The listing builds one solid part. Answer for the finished solid, in the listing's coordinates (mm). A direction names the side the tool comes from. Give positions to 0.01 mm unless a question says otherwise; leave off trailing zeros. Write each loop counter-clockwise with the first axis right and the second up, starting at its lowest first coordinate (ties: lowest second). Pieces come first, ordered by that corner, then holes. Notation, with made-up numbers: (-26, 79.25) - (-1, 79.25) arc R28 cw to (-1, 101.25) - close; hole circle Ø7 at (22.5, 24). An arc over 180 degrees is marked (long way). One line per item, written item: value. Start each with the question number.
Autodesk Inventor part; units mm, degrees
ref_plane "YZ Plane" through (0, 0, 0) normal (1, 0, 0) x (0, 1, 0)
ref_plane "XZ Plane" through (0, 0, 0) normal (0, 1, 0) x (-1, 0, 0)
ref_plane "XY Plane" through (0, 0, 0) normal (0, 0, 1) x (1, 0, 0)
sketch "Sketch1" plane through (0, 0, 0) normal (0, 0, 1) x (1, 0, 0)
  line L0 (127, 0) -> (127, 203.2)
  line L1 (127, 203.2) -> (0, 203.2)
  line L2 (0, 203.2) -> (0, 0)
  line L3 (95.25, 0) -> (95.25, 184.15)
  line L4 (95.25, 184.15) -> (31.75, 184.15)
  line L5 (31.75, 184.15) -> (31.75, 0)
  line L6 (0, 0) -> (31.75, 0)
  line L7 (95.25, 0) -> (127, 0)
  circle A0 centre (6.35, 6.35) radius 3.175
  circle A1 centre (120.65, 6.35) radius 3.175
  circle A2 centre (6.35, 196.85) radius 3.175
  circle A3 centre (120.65, 196.85) radius 3.175
  circle A4 centre (9.525, 101.6) radius 1.5875
  circle A5 centre (25.4, 101.6) radius 1.5875
  circle A6 centre (9.525, 76.2) radius 1.5875
  circle A7 centre (25.4, 76.2) radius 1.5875
extrude "Extrusion1" add sketch "Sketch1" along normal blind 15.875
chamfer "Chamfer1" distance 3.175 angle 45 2 edges at (31.75, 0, 7.9375) (95.25, 0, 7.9375)
fillet "Fillet1" radius 3.175 2 edges at (31.75, 184.15, 7.9375) (95.25, 184.15, 7.9375)
sketch "Sketch2" plane through (0, 0, 15.875) normal (0, 0, 1) x (1, 0, 0)
  arc A0 (6.35, 190.5) -> (12.7, 196.85) centre (6.35, 196.85) ccw
  line L0 (12.7, 196.85) -> (12.7, 203.2)
  line L1 (12.7, 203.2) -> (0, 203.2)
  line L2 (0, 203.2) -> (0, 190.5)
  line L3 (0, 190.5) -> (6.35, 190.5)
  arc A1 (114.3, 196.85) -> (120.65, 190.5) centre (120.65, 196.85) ccw
  line L4 (114.3, 196.85) -> (114.3, 203.2)
  line L5 (114.3, 203.2) -> (127, 203.2)
  line L6 (127, 203.2) -> (127, 190.5)
  line L7 (127, 190.5) -> (120.65, 190.5)
  arc A2 (12.7, 6.35) -> (6.35, 12.7) centre (6.35, 6.35) ccw
  line L8 (6.35, 12.7) -> (0, 12.7)
  line L9 (0, 12.7) -> (0, 0)
  line L10 (0, 0) -> (12.7, 0)
  line L11 (12.7, 0) -> (12.7, 6.35)
  arc A3 (120.65, 12.7) -> (114.3, 6.35) centre (120.65, 6.35) ccw
  line L12 (120.65, 12.7) -> (127, 12.7)
  line L13 (127, 12.7) -> (127, 0)
  line L14 (127, 0) -> (114.3, 0)
  line L15 (114.3, 0) -> (114.3, 6.35)
extrude "Extrusion2" cut sketch "Sketch2" against normal blind 5.5563
sketch "Sketch3" plane through (0, 0, 15.875) normal (0, 0, 1) x (1, 0, 0)
  line L0 (0, 93.6625) -> (31.75, 93.6625)
  line L1 (31.75, 93.6625) -> (31.75, 84.1375)
  line L2 (31.75, 84.1375) -> (0, 84.1375)
  line L3 (0, 84.1375) -> (0, 93.6625)
extrude "Extrusion3" cut sketch "Sketch3" against normal blind 12.7
properties part number "escapement base"
Item 1: Straight lines are drawn through the part: line 1 along Y through (x, z) = (25.4, 12.5); line 2 along X through (y, z) = (6.35, 4.25) (3 decimals); line 3 along X through (y, z) = (76.2, 8). For each, find the intervals that lie inside material, in ascending order.
Item 2: Find section A-A on y = 29.5. Determine the outline of the cut face in (x, z) (3 decimals).
Item 3: The mould has two halves that part along Y. Classify faces 1 (the flat face through (3, 5, 10.319)), 2 (the flat face through (14, 0, 6)), 3 (the flat face through (16, 93.662, 10)), 4 (the cylindrical face through (123.68, 5.4, 5.09)): +Y half, -Y half, draft (parallel to the pull), parting line (faces both ways), or undercut.
Item 4: For faces 5 (the flat face through (114.3, 200, 13)), 6 (the flat face through (124, 12.7, 13)), 7 (the flat face through (12.7, 3, 13)), determine the directions among +Z, -Z, +X, -X, +Y, -Y from which every point of the face is accessible in a straight line to the end or side of a thin tool.
Item 5: Find section B-B on x = 74.5. Determine the outline of the cut face in (y, z) (3 decimals), plus the area to 3 significant figures.
Item 6: Each of these flat-tipped pins is pushed along its axis until it touches: pin 1 Ø4.5 at (x, z) = (3.5, 12.5) entering from +Y; pin 2 Ø5 at (x, z) = (79.5, 8) entering from -Y; pin 3 Ø5 at (x, z) = (95.5, 11) entering from -Y (3 decimals); pin 4 Ø10 at (x, y) = (122.5, 7) entering from +Z. Where does it stop, or does it pass through?
Values:
1. line 1: 0 to 74.61, 77.79 to 84.14, 93.66 to 100.01, 103.19 to 203.2
1. line 2: 0 to 3.175, 9.525 to 31.75, 95.25 to 117.475, 123.825 to 127
1. line 3: 0 to 7.94, 11.11 to 23.81, 26.99 to 31.75, 95.25 to 127
2. outline: (0, 0) - (31.75, 0) - (31.75, 15.875) - (0, 15.875) - close; (95.25, 0) - (127, 0) - (127, 15.875) - (95.25, 15.875) - close
3. face 1: draft
3. face 2: -Y half
3. face 3: undercut
3. face 4: undercut
4. face 5: +Z, +X, +Y
4. face 6: +Z, +X, -Y
4. face 7: +Z, -X, -Y
5. outline: (184.15, 0) - (203.2, 0) - (203.2, 15.875) - (184.15, 15.875) - close
5. area: 302 mm^2
6. pin 1: y = 203.2
6. pin 2: y = 184.15
6. pin 3: y = 0.425
6. pin 4: z = 10.32
